Could you check a few things on this drawing? It's one solid part, dimensions in mm from its lowest x, y, z. A direction names the side the tool comes from. Round coordinates to 2 decimals unless told otherwise and drop trailing zeros. Loops run counter-clockwise (first coordinate to the right, second up) from the corner with the lowest first, then second, coordinate; pieces in that order, holes last.
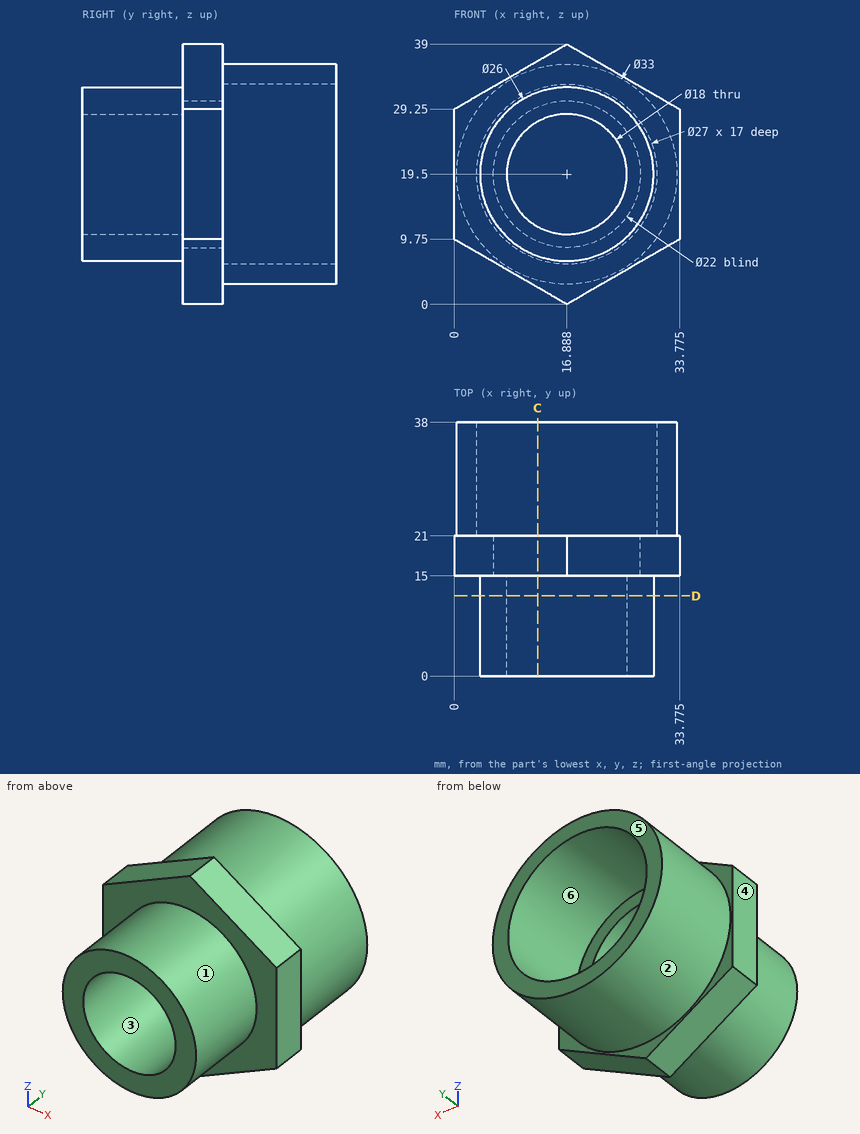
(1) Suppose I cut it at D-D (y = 12). Write out the boundary of the cut face in (x, z).
(2) For pin 1 (2 mm diameter, centred on y = 29, z = 18, fed in from -X) (1 decimal); pin 2 (6 mm diameter, centred on x = 5.5, y = 20.5, fed in from -Z), each with a flat end and sliding along its axis, tell me the tip position at first contact or that it passes through.
(3) Which directions (+Z, -Z, +X, -X, +Y, -Y) give clear straight access to the entire face, cutting with the end or side of a thin tool? Please do the marked faces 1, 2 and 3.
(4) If I drill on line 1 (X direction, y = 20, z = 20) (1 decimal); line 2 (X direction, y = 25, z = 19) (1 decimal); line 3 (Y direction, x = 28, z = 27.5), over which ranges is the centre line in solid material (lowest first)?
(5) We'd pull the mould along X, two halves only. Please class the marked faces 4, 5 and 6: released by +X, released by -X, zero draft, split by the parting line, or undercut.
(6) Suppose I cut it at C-C (x = 12.5). Write out the boundary of the cut face in (y, z) (1 decimal).
Check result:
1. outline: circle Ø26 at (16.89, 19.5); hole circle Ø18 at (16.89, 19.5)
2. pin 1: stops at x = 0.4
2. pin 2: stops at z = 4.84
3. face 1: -Y
3. face 2: +Y
3. face 3: +Y, -Y
4. line 1: x = 0 to 5.9, 27.9 to 33.8
4. line 2: x = 0.4 to 3.4, 30.4 to 33.4
4. line 3: y = 15 to 38
5. face 4: released by -X
5. face 5: zero draft
5. face 6: undercut
6. outline: (0, 7.3) - (15, 7.3) - (15, 2.5) - (21, 2.5) - (21, 3.6) - (38, 3.6) - (38, 6.7) - (21, 6.7) - (21, 9.4) - (15, 9.4) - (15, 11.6) - (0, 11.6) - close; (0, 27.4) - (15, 27.4) - (15, 29.6) - (21, 29.6) - (21, 32.3) - (38, 32.3) - (38, 35.4) - (21, 35.4) - (21, 36.5) - (15, 36.5) - (15, 31.7) - (0, 31.7) - close
